```python
from build123d import *

# Parameters (mm, degrees)
F0_R     = 2.875
F1_DEPTH = 20
F2_W     = 10
F2_H     = 14
F2_R     = 2.875
F3_DEPTH = 1.5
F4_R     = 5
F5_R     = 4.875
F5_R_2   = 2.875
F6_DEPTH = 1.75


with BuildPart() as f1:
    # F0 (on Top) → F1 (new body, symmetric)
    with BuildSketch(Plane.XY):
        Circle(F0_R)
    extrude(amount=F1_DEPTH, both=True)

    # F2 (on face) → F3 (join)
    with BuildSketch(Plane(origin=(0, 0, -20), x_dir=(1, 0, 0), z_dir=(0, 0, -1))):
        Rectangle(F2_W, F2_H)
        Circle(F2_R, mode=Mode.SUBTRACT)
        Circle(F2_R)
    extrude(amount=F3_DEPTH)

    # F4
    f4_edges = [f1.edges().sort_by_distance(p)[0] for p in [
        (-5, -7, -20.75),
        (5, 7, -20.75),
    ]]
    fillet(f4_edges, radius=F4_R)

    # F5 (on face) → F6 (join)
    with BuildSketch(Plane.XY.offset(-20)):
        Circle(F5_R)
        Circle(F5_R_2, mode=Mode.SUBTRACT)
    extrude(amount=F6_DEPTH)


solid = f1.part
```
CAD build for the part. Positions are in the model's coordinates, mm. A direction names the side the tool comes from. Round coordinates to 2 decimals unless told otherwise and drop trailing zeros. Write each loop counter-clockwise with the first axis right and the second up, starting at its lowest first coordinate (ties: lowest second). Pieces come first, ordered by that corner, then holes. Notation, with made-up numbers: (71.25, 25) -> (126.25, 25) arc R23 ccw to (126.25, 51) -> close; hole circle Ø6 at (9, 79.5). An arc over 180 degrees is marked (long way). Answer in a Markdown table with one row per item. Add a question column.
Item 1: Drill centre lines: line 1 (Z direction, x = 2.75, y = -5.5); line 2 (Z direction, x = 2.5, y = 3.5); line 3 (Y direction, x = 0, z = -14) (3 decimals). Where is each one in solid material? Low to high. Write a range as from..to.
Item 2: Drop flat-ended pins along their axis: pin 1 Ø5 at (y, z) = (-2.5, 10.5) entering from -X (3 decimals); pin 2 Ø8 at (y, z) = (0.5, 4.5) entering from +X (3 decimals); pin 3 Ø3 at (x, y) = (-0.5, 5.5) entering from +Z. Give the stop position or say it passes through.
Item 3: Saw through at C-C, the plane z = -0.5. Write the cut outline in (x, y) (3 decimals).
Item 4: Saw through at A-A, the plane y = 0. Write the cut outline in (x, z) (3 decimals), then the cut area to 3 significant figures.
Item 5: Which spindle directions (+Z, -Z, +X, -X, +Y, -Y) get a long thin tool onto all of the face, cutting with end or side? Do faces 1 (the face through (-0.635, 4.834, -19.137)), 2 (the face through (-5, 3, -21)). Say none if no direction does.
Item 6: Saw through at B-B, the plane x = 3.25. Write the cut outline in (y, z), then the cut area to 3 significant figures.
Item 7: Saw through at D-D, the plane y = -3.5. Write the cut outline in (x, z).
Item 8: Mould opens along Y. For faces 3 (the face through (-0.37, 2.85, 1.14)), 4 (the face through (0, 0, 20)), 5 (the face through (-4, -5, -21)) say: pulls with the +Y half, pulls with the -Y half, needs draft (parallel to the pull), parting line crosses it, or undercut.
Findings below:
| question | item | result |
|---|---|---|
| 1 | line 1 | z = -21.5..-20 |
| 1 | line 2 | z = -21.5..-18.25 |
| 1 | line 3 | y = -2.875..2.875 |
| 2 | pin 1 | stops at x = -2.875 |
| 2 | pin 2 | stops at x = 2.875 |
| 2 | pin 3 | stops at z = -18.25 |
| 3 | outline | circle Ø5.75 at (0, 0) |
| 4 | outline | (-5, -21.5) -> (5, -21.5) -> (5, -20) -> (4.875, -20) -> (4.875, -18.25) -> (2.875, -18.25) -> (2.875, 20) -> (-2.875, 20) -> (-2.875, -18.25) -> (-4.875, -18.25) -> (-4.875, -20) -> (-5, -20) -> close |
| 4 | area | 252 mm^2 |
| 5 | face 1 | +Z |
| 5 | face 2 | +Z, -Z, -X, +Y, -Y |
| 6 | outline | (-7, -21.5) -> (5.8, -21.5) -> (5.8, -20) -> (3.63, -20) -> (3.63, -18.25) -> (-3.63, -18.25) -> (-3.63, -20) -> (-7, -20) -> close |
| 6 | area | 31.9 mm^2 |
| 7 | outline | (-4.77, -21.5) -> (5, -21.5) -> (5, -20) -> (3.39, -20) -> (3.39, -18.25) -> (-3.39, -18.25) -> (-3.39, -20) -> (-4.77, -20) -> close |
| 8 | face 3 | parting line crosses it |
| 8 | face 4 | needs draft |
| 8 | face 5 | pulls with the -Y half |
